Geometry: see drawing. Coordinates: mm, zero at the bounding-box minimum. A direction names the side the tool comes from. Coordinates: 2 decimals unless noted, no trailing zeros. Order: outer loops, then holes, each group sorted by start corner. A loop starts at its lowest first (then second) coordinate and runs counter-clockwise, first axis right, second up.
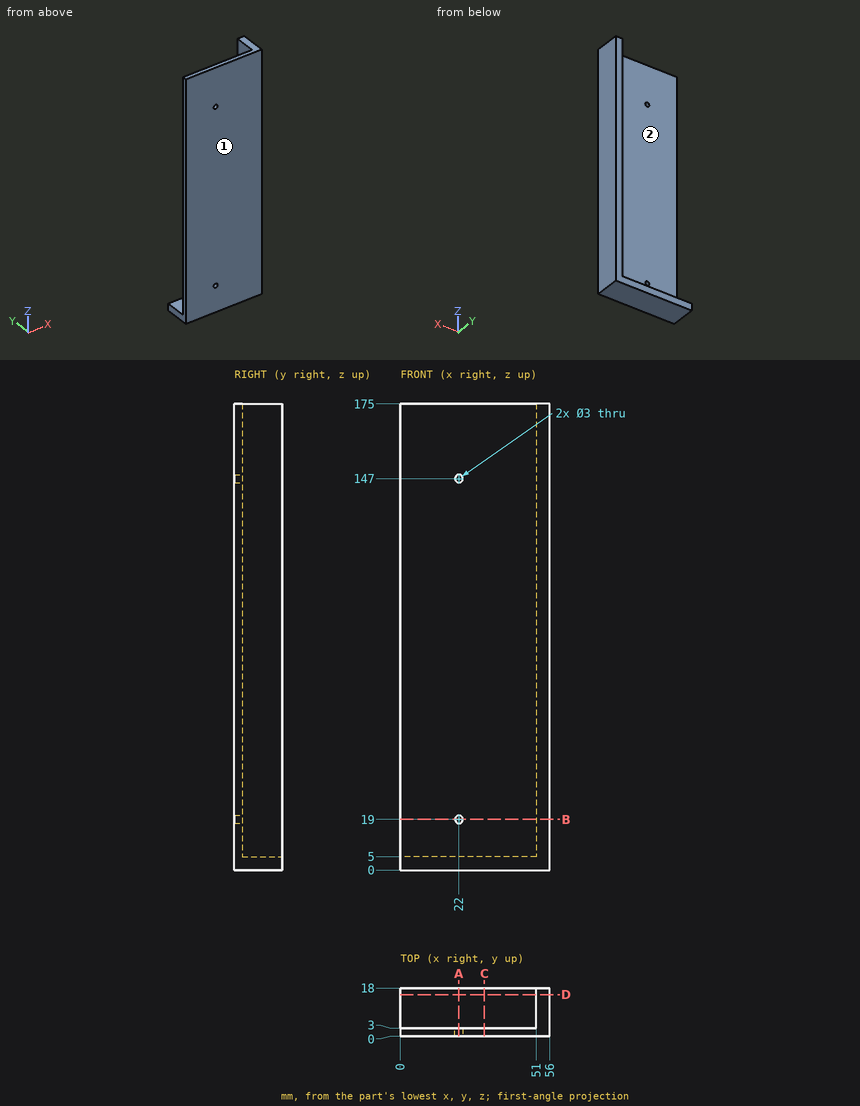
Item 1: Ray query, probe 1 along Z at (x, y) = (22, 2.05); probe 2 along Y at (x, z) = (9.5, 53); probe 3 along X at (y, z) = (12.75, 84). Return the intervals inside material, ascending.
Response values:
probe 1: z = 0 to 17.5, 20.5 to 145.5, 148.5 to 175
probe 2: y = 0 to 3
probe 3: x = 51 to 56
Item 2: Cut plane D-D on y = 15.5. Return loops of the section in (x, z), then the cut area to 3 significant figures.
Response values:
outline: (0, 0) - (56, 0) - (56, 175) - (51, 175) - (51, 5) - (0, 5) - close
area: 1,130 mm2
Item 3: Cut plane B-B on z = 19. Return loops of the section in (x, y).
Response values:
outline: (0, 0) - (20.5, 0) - (20.5, 3) - (0, 3) - close; (23.5, 0) - (56, 0) - (56, 18) - (51, 18) - (51, 3) - (23.5, 3) - close
Item 4: Access query for the marked faces 1 and 2. Directions: +Z, -Z, +X, -X, +Y, -Y. A direction counts if a zero-diameter tool reaches every point of the face in a straight line with its end or side. Return the directions, or none.
Response values:
face 1: +Z, -Z, +X, -X, -Y
face 2: +Z, -X, +Y
Item 5: Cut plane C-C on x = 31.5. Return loops of the section in (y, z), then the cut area to 3 significant figures.
Response values:
outline: (0, 0) - (18, 0) - (18, 5) - (3, 5) - (3, 175) - (0, 175) - close
area: 600 mm2
Item 6: Cut plane A-A on x = 22. Return loops of the section in (y, z).
Response values:
outline: (0, 0) - (18, 0) - (18, 5) - (3, 5) - (3, 17.5) - (0, 17.5) - close; (0, 20.5) - (3, 20.5) - (3, 145.5) - (0, 145.5) - close; (0, 148.5) - (3, 148.5) - (3, 175) - (0, 175) - close
Item 7: Pin query (flat end, axial travel): pin 1 Ø7.5 at (y, z) = (7, 79) entering from -X; pin 2 Ø3.5 at (x, z) = (22, 19) entering from +Y. Return the tip coordinate at first contact, or that it passes through.
Response values:
pin 1: stops at x = 51
pin 2: stops at y = 3
